from build123d import *

# Parameters (mm, degrees)
CIRPATTERN1_COUNT = 2
CIRPATTERN1_ANGLE = 90


# Read off the part's stored shape, not the designer's step: ThreadSchematic
with BuildPart() as part:
    # ThreadSchematic outline → ThreadSchematic (revolve)
    with BuildSketch(Plane.YX):
        with BuildLine():
            Line((0, 14.6812), (0, 0))
            ThreePointArc((0, 0), (1.546391238, 0.560330696), (2.3749, 1.981200001))
            Line((2.3749, 1.981200001), (1.2573, 1.9812))
            Line((1.2573, 1.9812), (1.2573, 14.6812))
            Line((1.2573, 14.6812), (0, 14.6812))
        make_face()
    revolve(axis=Axis((0, 0, 0), (1, 0, 0)))

    # Sketch3 → Cross section 0
    with BuildSketch(Plane(origin=(0, 0, 0), x_dir=(0, 0, -1), z_dir=(1, 0, 0))):
        with BuildLine():
            Line((0.3429, -1.5494), (-0.3429, -1.5494))
            Line((-0.3429, -1.5494), (-0.3429, 1.5494))
            Line((-0.3429, 1.5494), (0.3429, 1.5494))
            Line((0.3429, 1.5494), (0.3429, -1.5494))
        make_face()
    # Sketch4 → Cross section 1
    with BuildSketch(Plane(origin=(1.7018, 0, 0), x_dir=(0, 0, -1), z_dir=(1, 0, 0))):
        with BuildLine():
            Line((0.17145, -0.17145), (-0.17145, -0.17145))
            Line((-0.17145, -0.17145), (-0.17145, 0.17145))
            Line((-0.17145, 0.17145), (0.17145, 0.17145))
            Line((0.17145, 0.17145), (0.17145, -0.17145))
        make_face()
    cross = loft(mode=Mode.SUBTRACT)

    # CirPattern1: Cross ×2 about axis
    cirpattern1_axis = Axis((0, 0, 0), (1, 0, 0))
    for i in range(1, CIRPATTERN1_COUNT):
        add(cross.rotate(cirpattern1_axis, i * CIRPATTERN1_ANGLE / (CIRPATTERN1_COUNT - 1)), mode=Mode.SUBTRACT)


solid = part.part
Part model, mm, in its own coordinate system. A direction names the side the tool comes from. Coordinates: 2 decimals unless noted, no trailing zeros. Loops run counter-clockwise (first coordinate to the right, second up) from the corner with the lowest first, then second, coordinate; pieces in that order, holes last. Notation, with made-up numbers: M -2.5,38 L 56.5,38 A18 ccw 56.5,56 Z; hole C -25.75,-33.75 d7. An arc over 180 degrees is marked long. Use a Markdown table: item, result. Add a question column.
Q1. Pin check, flat tips, straight feed: P1, Ø1.5, axis at x = 8.5, z = 1.5, coming from the -Y side; P2, Ø1.5, axis at y = -0.5, z = 0, coming from the -X side; P3, Ø2, axis at y = 2, z = -1.5, coming from the +X side; P4, Ø2, axis at x = 8, y = -0.5, coming from the -Z side. Stop position of each tip, or through.
Q2. Cut at B-B (z = 1.5). Write the cut outline in (x, y).
Q3. Which spindle directions (+Z, -Z, +X, -X, +Y, -Y) get a long thin tool onto all of the face, cutting with end or side? Do faces 1 (the flat face through (1.981, 1, -1)), 2 (the flat face through (14.681, 0, 0)). Say none if no direction does.
Q4. Cut at A-A (x = 9.75). Write the cut outline in (y, z).
Q5. Probe L1, parallel to Y at x = 6.75, z = -0.1; L2, parallel to Z at x = 8, y = -0.05; L3, parallel to Y at x = 13, z = 0.5. List the from-to ranges inside material, lowest first.
Worked out:
| question | item | result |
|---|---|---|
| 1 | P1 | stops at y = -1.01 |
| 1 | P2 | stops at x = 0.05 |
| 1 | P3 | stops at x = 1.98 |
| 1 | P4 | stops at z = -1.26 |
| 2 | outline | M 1.98,-1.84 L 1.98,1.84 A1.89 ccw Z |
| 3 | face 1 | +X |
| 3 | face 2 | +Z, -Z, +X, +Y, -Y |
| 4 | outline | C 0,0 d2.51 |
| 5 | L1 | y = -1.25 to 1.25 |
| 5 | L2 | z = -1.26 to 1.26 |
| 5 | L3 | y = -1.15 to 1.15 |
